```python
from build123d import *

# Parameters (mm, degrees)
BOSS_EXTRUDE1_DEPTH = 6
SKETCH2_R           = 462.5
CUT_EXTRUDE1_DEPTH  = 10
SKETCH3_R           = 4
CUT_EXTRUDE2_DEPTH  = 10
CIRPATTERN1_COUNT   = 16
FILLET1_R           = 6


with BuildPart() as part:
    # Sketch1 → Boss-Extrude1 (new body)
    with BuildSketch(Plane(origin=(0, 0, 0), x_dir=(1, 0, 0), z_dir=(0, 1, 0))):
        Polygon((315.066450454, 496.5), (497.5, 314.066450454), (497.5, -315.066450454), (315.066450454, -497.5), (-314.066450454, -497.5), (-496.5, -315.066450454), (-496.5, 314.066450454), (-314.066450454, 496.5), align=None)
    extrude(amount=BOSS_EXTRUDE1_DEPTH)

    # Sketch2 → Cut-Extrude1 (cut)
    with BuildSketch(Plane(origin=(0, 6, 0), x_dir=(1, 0, 0), z_dir=(0, 1, 0))):
        with Locations(Location((0, 0, 0), (0, 0, 270))):
            Circle(SKETCH2_R)
    extrude(amount=-CUT_EXTRUDE1_DEPTH, mode=Mode.SUBTRACT)

    # Sketch3 → Cut-Extrude2 (cut)
    with BuildSketch(Plane(origin=(0, 6, 0), x_dir=(1, 0, 0), z_dir=(0, 1, 0))):
        with Locations(Location((0, 480, 0), (0, 0, 270))):
            Circle(SKETCH3_R)
    cut_extrude2 = extrude(amount=-CUT_EXTRUDE2_DEPTH, mode=Mode.SUBTRACT)

    # CirPattern1: Cut-Extrude2 ×16 about axis
    cirpattern1_axis = Axis((0, 0, 0), (0, 1, 0))
    for i in range(1, CIRPATTERN1_COUNT):
        add(cut_extrude2.rotate(cirpattern1_axis, i * 360 / CIRPATTERN1_COUNT), mode=Mode.SUBTRACT)

    # Fillet1
    fillet1_edges = [part.edges().sort_by_distance(p)[0] for p in [
        (315.066450454, 3, -496.5),
        (497.5, 3, -314.066450454),
        (497.5, 3, 315.066450454),
        (315.066450454, 3, 497.5),
        (-314.066450454, 3, 497.5),
        (-496.5, 3, 315.066450454),
        (-496.5, 3, -314.066450454),
        (-314.066450454, 3, -496.5),
    ]]
    fillet(fillet1_edges, radius=FILLET1_R)


solid = part.part
```
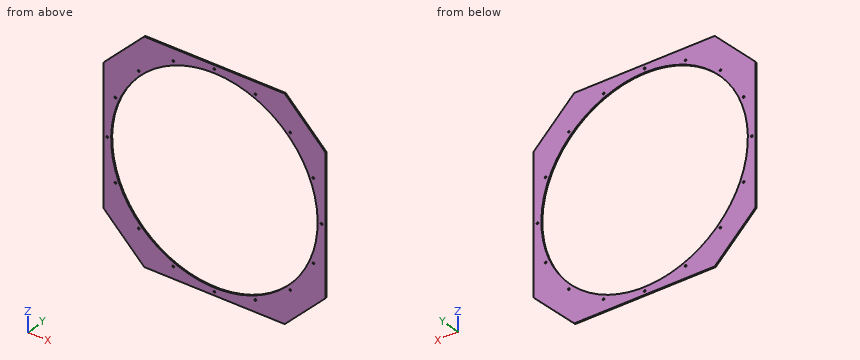
Verification items for the finished model (mm, model axes). Give positions to 0.01 mm unless a question says otherwise; leave off trailing zeros. Order: outer loops, then holes, each group sorted by start corner. A loop starts at its lowest first (then second) coordinate and runs counter-clockwise, first axis right, second up. Notation, with made-up numbers: M 31.5,41.25 L 60.5,41.25 A25 cw 60.5,75.25 Z; hole C -7,8.25 d8. An arc over 180 degrees is marked long. Answer in a Markdown table with one row per item. Add a question column.
Item 1: Section check B-B, the plane z = -138. Enter the section's corners in (x, y).
Item 2: Section check A-A, the plane x = -388. Enter the section's corners in (y, z), and give its area (3 significant figures).
Item 3: Scan lines: probe 1 along X at (y, z) = (2.1, -66); probe 2 along X at (y, z) = (3.9, -150.5); probe 3 along Z at (x, y) = (36.5, 5.3). Record each from-to range of solid material in increasing order. Write a range as from..to.
Item 4: Section check C-C, the plane y = 2.55. State how many separate pieces and enclosed holes the cut face has, and give its area (3 significant figures).
Item 5: Gauge pin test, flat end, axial feed: pin 1 (10.5 mm diameter, centred on x = 0, z = 480, fed in from -Y). Record the tip position at first contact, or that the pin passes through.
Filled sheet:
| question | item | result |
|---|---|---|
| 1 | outline | M -496.5,0 L -441.43,0 L -441.43,6 L -496.5,6 Z; M 441.43,0 L 497.5,0 L 497.5,6 L 441.43,6 Z |
| 2 | outline | M 0,-422.57 L 6,-422.57 L 6,-251.72 L 0,-251.72 Z; M 0,251.72 L 6,251.72 L 6,423.57 L 0,423.57 Z |
| 2 | area | 2,060 mm^2 |
| 3 | probe 1 | x = -496.5..-457.77, 457.77..497.5 |
| 3 | probe 2 | x = -496.5..-437.33, 437.33..497.5 |
| 3 | probe 3 | z = -496.5..-461.06, 461.06..497.5 |
| 4 | separate pieces | 1 |
| 4 | enclosed holes | 17 |
| 4 | area | 249,000 mm^2 |
| 5 | pin 1 | stops at y = 0 |
